from build123d import *

# Parameters (mm, degrees)
F1_DEPTH = 3.1242
F2_R     = 1.5875
F3_DEPTH = 34.925
F4_R     = 0.635
F5_DEPTH = 5.6642


with BuildPart() as f1:
    # F0 (on Front) → F1 (new body)
    with BuildSketch(Plane.XZ):
        Polygon((0.125082, 23.970308), (0, 25.4), (-6.083153, 23.185914), (-6.574004, 24.534516), (-11.87683, 20.821437), (-12.7, 21.997045), (-16.861121, 17.038014), (-17.960512, 17.960512), (-20.696355, 12.093478), (-21.997045, 12.7), (-23.121166, 6.324792), (-24.534516, 6.574004), (-23.970308, 0.125082), (-25.4, 0), (-23.185914, -6.083153), (-24.534516, -6.574004), (-20.821437, -11.87683), (-21.997045, -12.7), (-17.038014, -16.861121), (-17.960512, -17.960512), (-12.093478, -20.696355), (-12.7, -21.997045), (-6.324792, -23.121166), (-6.574004, -24.534516), (-0.125082, -23.970308), (0, -25.4), (6.083153, -23.185914), (6.574004, -24.534516), (11.87683, -20.821437), (12.7, -21.997045), (16.861121, -17.038014), (17.960512, -17.960512), (20.696355, -12.093478), (21.997045, -12.7), (23.121166, -6.324792), (24.534516, -6.574004), (23.970308, -0.125082), (25.4, 0), (23.185914, 6.083153), (24.534516, 6.574004), (20.821437, 11.87683), (21.997045, 12.7), (17.038014, 16.861121), (17.960512, 17.960512), (12.093478, 20.696355), (12.7, 21.997045), (6.324792, 23.121166), (6.574004, 24.534516), align=None)
    extrude(amount=F1_DEPTH)

    # F2 (on face) → F3 (join)
    with BuildSketch(Plane(origin=(0, 0, 0), x_dir=(-1, 0, 0), z_dir=(0, 1, 0))):
        Circle(F2_R)
    extrude(amount=F3_DEPTH)

    # F4 (on face) → F5 (join)
    with BuildSketch(Plane(origin=(0, 34.925, 0), x_dir=(-1, 0, 0), z_dir=(0, 1, 0))):
        Circle(F4_R)
    extrude(amount=F5_DEPTH)


solid = f1.part
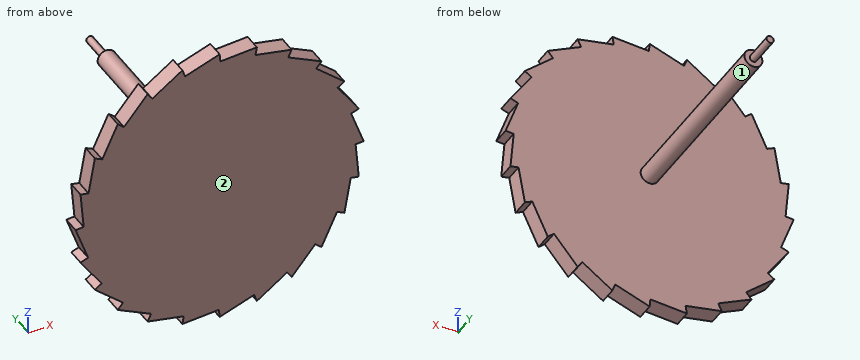
The listing builds one solid part. Answer for the finished solid, in the listing's coordinates (mm). Face numbers are marked on the shaded views. A direction names the side the tool comes from. Give positions to 0.01 mm unless a question says otherwise; leave off trailing zeros. Write each loop counter-clockwise with the first axis right and the second up, starting at its lowest first coordinate (ties: lowest second). Pieces come first, ordered by that corner, then holes.
Item 1: Section B-B, the plane z = -4 is taken. Write down the section's boundary in (x, y).
Item 2: Which of the six approach directions +Z, -Z, +X, -X, +Y, -Y give full straight-line access (tool end or side, diameter ignored) to the marked faces 1 and 2?
Item 3: Find the intervals of material crossed by line 1 along Y through (x, z) = (-8.5, -7); line 2 along X through (y, z) = (11, 1), in increasing order.
Item 4: Flat-ended cylindrical pins translate along their axes: P1, Ø1, axis at x = 1.5, y = 9, coming from the -Z side; P2, Ø4, axis at x = -0.5, y = 19, coming from the -Z side; P3, Ø1, axis at x = 8, z = 1.5, coming from the +Y side. Find the tip coordinate at first contact, or state that the pin passes through.
Item 5: Section A-A, the plane y = 15 is taken. Write down the section's boundary in (x, z) (1 decimal).
Completed:
1. outline: (-23.94, -3.12) - (24.31, -3.12) - (24.31, 0) - (-23.94, 0) - close
2. face 1: +Y
2. face 2: +Z, -Z, +X, -X, -Y
3. line 1: y = -3.12 to 0
3. line 2: x = -1.23 to 1.23
4. P1: stops at z = -1.23
4. P2: stops at z = -1.59
4. P3: stops at y = 0
5. outline: circle Ø3.2 at (0, 0)
